Here's the drawing with two shaded views (mm, measured from the low corner). I have some questions. A direction names the side the tool comes from. Round coordinates to 2 decimals unless told otherwise and drop trailing zeros. Order: outer loops, then holes, each group sorted by start corner. A loop starts at its lowest first (then second) coordinate and runs counter-clockwise, first axis right, second up.
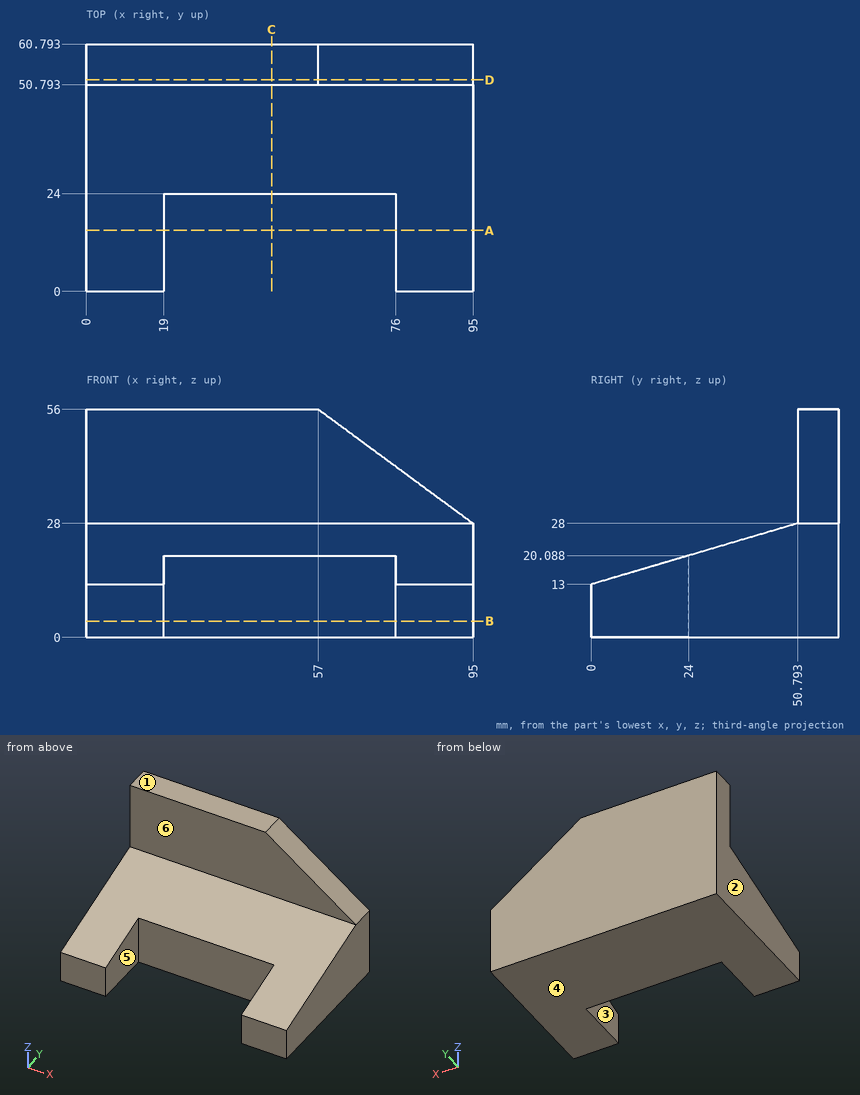
1. On a 3-axis mill with a long thin cutter (end or side, diameter ignored), from which of +Z, -Z, +X, -X, +Y, -Y can I reach the whole of each face in a straight line? I mean the marked faces 4, 5 and 6. Say none if no direction works.
Evaluation:
face 4: -Z, +X, -X, +Y, -Y
face 5: +Z, -Z, -Y
face 6: +Z, +X, -X, -Y
2. If we mould it in two halves opening along X, with no side actions, what happens to the marked faces 1, 2 and 3? For each: released by +X, released by -X, zero draft, split by the parting line, or undercut.
Evaluation:
face 1: zero draft
face 2: released by -X
face 3: undercut
3. If we section it at D-D, the plane y = 52: Write out the boundary of the cut face in (x, z), and give its area (3 significant figures).
Evaluation:
outline: (0, 0) - (95, 0) - (95, 28) - (57, 56) - (0, 56) - close
area: 4,790 mm2
4. I'm going to push flat-ended pins straight in: P1, Ø4, axis at x = 30.5, z = 33.5, coming from the -Y side; P2, Ø6, axis at x = 41.5, z = 7.5, coming from the -Y side; P3, Ø1.5, axis at x = 74, y = 18, coming from the -Z side. Where does each tip first touch, or does it pass through?
Evaluation:
P1: stops at y = 50.79
P2: stops at y = 24
P3: passes through
5. I need wall thicknesses on probe 1 along Y at (x, z) = (21, 32); probe 2 along X at (y, z) = (21.5, 12); probe 3 along Y at (x, z) = (64, 19). Which ranges of each line are inside material? Lowest first, please.
Evaluation:
probe 1: y = 50.79 to 60.79
probe 2: x = 0 to 19, 76 to 95
probe 3: y = 24 to 60.79
6. If we section it at A-A, the plane y = 15: Write out the boundary of the cut face in (x, z), and give its area (3 significant figures).
Evaluation:
outline: (0, 0) - (19, 0) - (19, 17.43) - (0, 17.43) - close; (76, 0) - (95, 0) - (95, 17.43) - (76, 17.43) - close
area: 662 mm2
7. If we section it at B-B, the plane z = 4: Write out the boundary of the cut face in (x, y).
Evaluation:
outline: (0, 0) - (19, 0) - (19, 24) - (76, 24) - (76, 0) - (95, 0) - (95, 60.79) - (0, 60.79) - close
8. If we section it at C-C, the plane x = 45.5: Write out the boundary of the cut face in (y, z).
Evaluation:
outline: (24, 0) - (60.79, 0) - (60.79, 56) - (50.79, 56) - (50.79, 28) - (24, 20.09) - close
